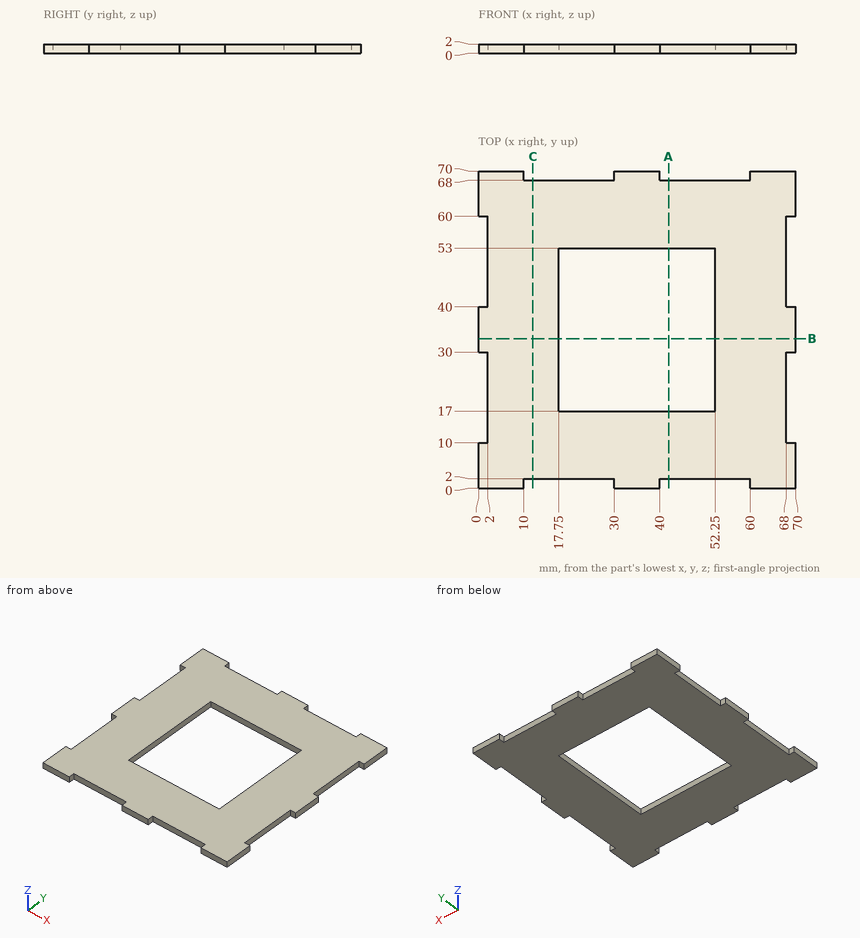
Check sheet for the drawn part. Datum: minimum x, y, z corner. Units: mm. Give positions to 0.01 mm unless a question says otherwise; leave off trailing zeros. Loops run counter-clockwise (first coordinate to the right, second up) from the corner with the lowest first, then second, coordinate; pieces in that order, holes last.
1) Sectioned sample at B-B, the plane y = 33. Enter the section's corners in (x, z), then the cut area to 3 significant figures.
2) Sectioned sample at A-A, the plane x = 42. Enter the section's corners in (y, z), then the cut area to 3 significant figures.
3) Sectioned sample at C-C, the plane x = 12. Enter the section's corners in (y, z).
4) Thickness scan on line 1 along X through (y, z) = (34, 1.4); line 2 along Y through (x, z) = (24, 1.4); line 3 along X through (y, z) = (49, 0.45). Record the ranges inside material, lowest first.
5) Depth check by flat-ended pin: pin 1 Ø0.6 at (y, z) = (22.5, 1) entering from +X; pin 2 Ø1 at (y, z) = (23.5, 1.5) entering from -X; pin 3 Ø1 at (x, z) = (52, 0.5) entering from +Y. Enter the tip coordinate at first touch or a pass-through.
Answers:
1. outline: (0, 0) - (17.75, 0) - (17.75, 2) - (0, 2) - close; (52.25, 0) - (70, 0) - (70, 2) - (52.25, 2) - close
1. area: 71.0 mm2
2. outline: (2, 0) - (17, 0) - (17, 2) - (2, 2) - close; (53, 0) - (68, 0) - (68, 2) - (53, 2) - close
2. area: 60.0 mm2
3. outline: (2, 0) - (68, 0) - (68, 2) - (2, 2) - close
4. line 1: x = 0 to 17.75, 52.25 to 70
4. line 2: y = 2 to 17, 53 to 68
4. line 3: x = 2 to 17.75, 52.25 to 68
5. pin 1: stops at x = 68
5. pin 2: stops at x = 2
5. pin 3: stops at y = 68
